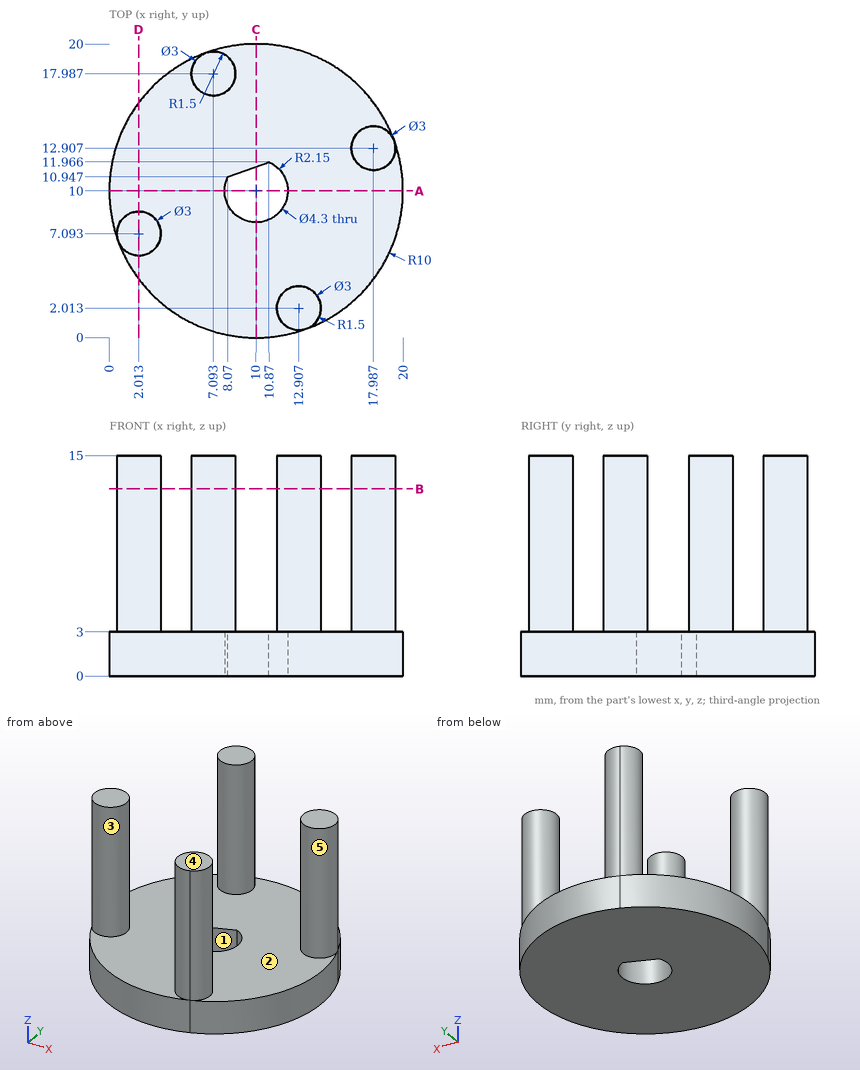
Verification items for this drawing (mm, ordinates from the low corner). A direction names the side the tool comes from. Round coordinates to 2 decimals unless told otherwise and drop trailing zeros. Order: outer loops, then holes, each group sorted by start corner. A loop starts at its lowest first (then second) coordinate and runs counter-clockwise, first axis right, second up. Notation, with made-up numbers: (3.5, 57) -> (24.5, 57) arc R26 ccw to (24.5, 88) -> close; hole circle Ø5 at (13.5, 32.5). An arc over 180 degrees is marked (long way). Use one line per item in the form item = value.
1. Mould release check, pull along Y, two halves, no side actions. Record for the marked faces 1, 2 and 3: pulls with the +Y half, pulls with the -Y half, needs draft (parallel to the pull), parting line crosses it, or undercut.
Working result:
face_1 = undercut
face_2 = needs draft
face_3 = parting line crosses it
2. Cross-section at B-B, the plane z = 12.75. Enter the section's corners in (x, y) (1 decimal).
Working result:
outline = circle Ø3 at (2, 7.1); circle Ø3 at (7.1, 18); circle Ø3 at (12.9, 2); circle Ø3 at (18, 12.9)
3. Scan lines: line 1 along X through (y, z) = (10, 0.9); line 2 along Y through (x, z) = (10, 2.05); line 3 along Y through (x, z) = (9.5, 1). Record each from-to range of solid material in increasing order. Write a range as from..to.
Working result:
line_1 = 0..7.85, 12.15..20
line_2 = 0..7.85, 11.65..20
line_3 = 0.01..7.91, 11.47..19.99
4. Set-up check for the marked faces 4 and 5: record each of +Z, -Z, +X, -X, +Y, -Y from which the full face is reachable in a straight line by a thin tool's end or side.
Working result:
face_4 = +Z, +X, -X, +Y, -Y
face_5 = +Z
5. Go/stop test with flat-tipped pins: pin 1 (4 mm diameter, centred on x = 9, z = 11.5, fed in from +Y); pin 2 (5.5 mm diameter, centred on x = 10, y = 10, fed in from +Z); pin 3 (8 mm diameter, centred on y = 16, z = 7.5, fed in from -X); pin 4 (1 mm diameter, centred on x = 15, z = 4, fed in from -Y). Record where each tip stops, or that it passes through.
Working result:
pin_1 = 19.49
pin_2 = 3
pin_3 = 5.59
pin_4 = through
6. Cross-section at D-D, the plane x = 2. Enter the section's corners in (y, z).
Working result:
outline = (4, 0) -> (16, 0) -> (16, 3) -> (8.59, 3) -> (8.59, 15) -> (5.59, 15) -> (5.59, 3) -> (4, 3) -> close
7. Cross-section at C-C, the plane x = 10. Enter the section's corners in (y, z).
Working result:
outline = (0, 0) -> (7.85, 0) -> (7.85, 3) -> (0, 3) -> close; (11.65, 0) -> (20, 0) -> (20, 3) -> (11.65, 3) -> close
8. Cross-section at A-A, the plane y = 10. Enter the section's corners in (x, z).
Working result:
outline = (0, 0) -> (7.85, 0) -> (7.85, 3) -> (0, 3) -> close; (12.15, 0) -> (20, 0) -> (20, 3) -> (12.15, 3) -> close
